Read the model definition and answer for the solid it produces. Units are mm, in the model's axes. A direction names the side the tool comes from. Coordinates: 2 decimals unless noted, no trailing zeros. Order: outer loops, then holes, each group sorted by start corner. A loop starts at its lowest first (then second) coordinate and runs counter-clockwise, first axis right, second up. Notation, with made-up numbers: (52.25, -17) - (81.25, -17) arc R10 cw to (81.25, -3) - close; hole circle Ø5 at (-38.75, 13). An arc over 180 degrees is marked (long way). Use one line per item in the form item = value.
Autodesk Inventor part; units mm, degrees
ref_plane "YZ Plane" through (0, 0, 0) normal (1, 0, 0) x (0, 1, 0)
ref_plane "XZ Plane" through (0, 0, 0) normal (0, 1, 0) x (-1, 0, 0)
ref_plane "XY Plane" through (0, 0, 0) normal (0, 0, 1) x (1, 0, 0)
sketch "Sketch1" plane through (0, 0, 0) normal (0, 0, 1) x (1, 0, 0)
  line L0 (-9.9228, -35) -> (-13.5328, -35)
  line L1 (-13.5328, -35) -> (-13.5328, -31)
  line L2 (-13.5328, -31) -> (-9.9228, -31)
  line L3 (-9.9228, -31) -> (-9.9228, -35)
  line L4 (-9.9228, -35) -> (-9.9228, -55)
  line L5 (-9.9228, -55) -> (-11.9228, -55)
  line L6 (-11.9228, -55) -> (-11.9228, -35)
  point P0 (0, 0)
  dimension "d0" = 3.61
  dimension "d1" = 4
  dimension "d3" = 2
  dimension "d16" = 20
revolve "Revolution1" add sketch "Sketch1" angle 360 about axis through (-9.9228, -35, 0) along (0, -1, 0)
chamfer "Chamfer1" distance 0.4 angle 45 1 edges at (-6.3128, -31, 0)
sketch "Boceto2" plane through (-9.9228, -31, 0) normal (0, 1, 0) x (1, 0, 0)
  line L0 (1.1641, -1.3443) -> (-0.5821, -1.6803)
  line L1 (-0.5821, -1.6803) -> (-1.7462, -0.336)
  line L2 (-1.7462, -0.336) -> (-1.1641, 1.3443)
  line L3 (-1.1641, 1.3443) -> (0.5821, 1.6803)
  line L4 (0.5821, 1.6803) -> (1.7462, 0.336)
  line L5 (1.7462, 0.336) -> (1.1641, -1.3443)
  point P0 (9.9228, 0)
  point P1 (0, 0)
  dimension "d11" = 3.08
extrude "Extrusión1" cut sketch "Boceto2" against normal blind 2
thread "Rosca1"
properties part number "Tornillo Allen cabeza cilindrica M4x20mm"
(1) Section B-B, the plane z = 0 is taken. Write down the section's boundary in (x, y), then the cut area to 3 significant figures.
Answer list:
outline = (-13.53, -35) - (-11.92, -35) - (-11.92, -55) - (-7.92, -55) - (-7.92, -35) - (-6.31, -35) - (-6.31, -31.4) - (-6.71, -31) - (-8.29, -31) - (-8.29, -33) - (-11.55, -33) - (-11.55, -31) - (-13.13, -31) - (-13.53, -31.4) - close
area = 102 mm2
(2) Given pin 1 Ø1 at (x, z) = (-10, 0) entering from +Y; pin 2 Ø1.5 at (y, z) = (-38.5, 1.5) entering from +X; pin 3 Ø4 at (y, z) = (-43, -1) entering from -X, each flat-ended and moving along its own axis, determine where each tip first touches the part or whether it passes through.
Answer list:
pin_1 = -33
pin_2 = -8.07
pin_3 = -11.92
(3) Section A-A, the plane y = -44.5 is taken. Write down the section's boundary in (x, z), then the cut area to 3 significant figures.
Answer list:
outline = circle Ø4 at (-9.92, 0)
area = 12.6 mm2
(4) Which of the six approach directions +Z, -Z, +X, -X, +Y, -Y give full straight-line access (tool end or side, diameter ignored) to faces 1 (the flat face through (-11, -35, 2)), 2 (the flat face through (-8, -31, 1)), 3 (the flat face through (-11.079, -31.986, 1.018))?
Answer list:
face_1 = -Y
face_2 = +Z, -Z, +X, -X, +Y
face_3 = +Y
(5) The mould has two halves that part along Z. Classify faces 4 (the flat face through (-10, -33, 0)), 5 (the cylindrical face through (-6.316, -33.175, 0.159)), 6 (the flat face through (-10, -55, 0)): +Z half, -Z half, draft (parallel to the pull), parting line (faces both ways), or undercut.
Answer list:
face_4 = undercut
face_5 = parting line
face_6 = draft
(6) Straight lines are drawn through the part: L1, parallel to Y at x = -8, z = -2; L2, parallel to Z at x = -11, y = -53.75; L3, parallel to X at y = -39.25, z = 0. For each, find the intervals that lie inside material, in ascending order.
Answer list:
L1 = -35 to -31
L2 = -1.69 to 1.69
L3 = -11.92 to -7.92
